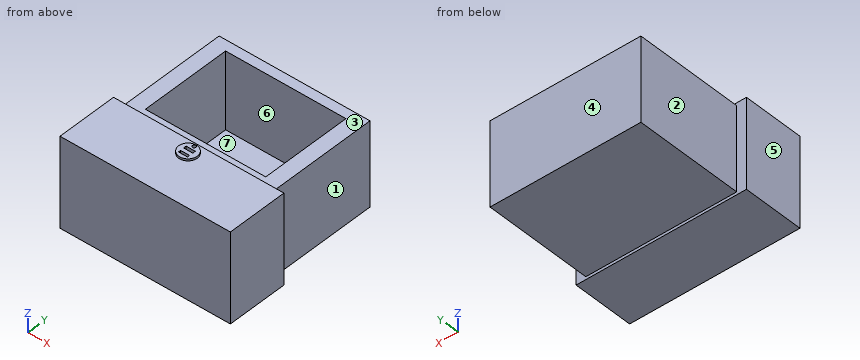
from build123d import *

# Parameters (mm, degrees)
F0_W      = 236.721322
F0_H      = 124.82763
F1_DEPTH  = 84.582
F2_W      = 209.650278
F2_H      = 117.007106
F3_DEPTH  = 151.384
F4_W      = 167.194322
F4_H      = 126.676479
F5_DEPTH  = 106.934
F6_R      = 12.932429
F7_DEPTH  = 2.794
F8_W      = 12.893153
F8_H      = 4.004114
F8_W_2    = 12.566442
F8_H_2    = 3.328527
F9_DEPTH  = 14.732
F10_R     = 2.422057
F11_DEPTH = 25.4


with BuildPart() as f1:
    # F0 (on Front) → F1 (new body)
    with BuildSketch(Plane.XZ):
        Rectangle(F0_W, F0_H)
    extrude(amount=F1_DEPTH)

    # F2 (on face) → F3 (join)
    with BuildSketch(Plane(origin=(0, 0, 0), x_dir=(-1, 0, 0), z_dir=(0, 1, 0))):
        Rectangle(F2_W, F2_H)
    extrude(amount=F3_DEPTH)

    # F4 (on face) → F5 (cut)
    with BuildSketch(Plane.XY.offset(58.503553)):
        with Locations((0, 74.151702)):
            Rectangle(F4_W, F4_H)
    extrude(amount=-F5_DEPTH, mode=Mode.SUBTRACT)

    # F6 (on face) → F7 (join)
    with BuildSketch(Plane.XY.offset(62.413815)):
        with Locations((0, -16.961597)):
            Circle(F6_R)
    extrude(amount=F7_DEPTH)

    # F8 (on face) → F9 (cut)
    with BuildSketch(Plane.XY.offset(65.207815)):
        with Locations((-0.298541, -14.347668)):
            Rectangle(F8_W, F8_H)
        with Locations((-0.135185, -23.072623)):
            Rectangle(F8_W_2, F8_H_2)
    extrude(amount=-F9_DEPTH, mode=Mode.SUBTRACT)

    # F10 (on face) → F11 (cut)
    with BuildSketch(Plane.XY.offset(65.207815)):
        with Locations((0, -7.139143)):
            Circle(F10_R)
    extrude(amount=-F11_DEPTH, mode=Mode.SUBTRACT)


solid = f1.part
Could you check a few things on this model? Use its own coordinates, in mm. Face numbers are marked on the shaded views. A direction names the side the tool comes from. Give positions to 0.01 mm unless a question says otherwise; leave off trailing zeros. Write each loop counter-clockwise with the first axis right and the second up, starting at its lowest first coordinate (ties: lowest second). Pieces come first, ordered by that corner, then holes. Notation, with made-up numbers: (-28, -5) -> (9, -5) arc R18 cw to (9, 19) -> close; hole circle Ø8 at (59, 26.5). An arc over 180 degrees is marked (long way). Answer as CSV lines item,"result". Start each with the question number.
(1) If we mould it in two halves opening along Y, with no side actions, what happens to the marked faces 4, 5, 6 and 7? For each: +Y half, -Y half, draft (parallel to the pull), parting line (faces both ways), or undercut.
(2) If we section it at A-A, the plane z = 20.5: Write out the boundary of the cut face in (x, y).
(3) Which directions (+Z, -Z, +X, -X, +Y, -Y) give clear straight access to the entire face, cutting with the end or side of a thin tool? Please do the marked faces 1, 2 and 3.
(4) I'm going to push flat-ended pins straight in: pin 1 Ø1.5 at (y, z) = (36.5, 16) entering from -X; pin 2 Ø4 at (x, y) = (48.5, 81) entering from +Z; pin 3 Ø2.5 at (x, y) = (1, -7.5) entering from +Z. Where does each tip first touch, or does it pass through?
(5) If we section it at B-B, the plane x = 31: Write out the boundary of the cut face in (y, z), and give its area (3 significant figures).
(6) Please list where these lines run through material, in increasing order: line 1 (Y direction, x = 0, z = 55); line 2 (X direction, y = 121.5, z = 31.5); line 3 (Y direction, x = 8.5, z = 18).
(7) If we section it at C-C, the plane y = 114.5: Write out the boundary of the cut face in (x, z), and give its area (3 significant figures).
Answer list:
1,face 4,"+Y half"
1,face 5,"draft"
1,face 6,"undercut"
1,face 7,"undercut"
2,outline,"(-118.36, -84.58) -> (118.36, -84.58) -> (118.36, 0) -> (104.83, 0) -> (104.83, 151.38) -> (-104.83, 151.38) -> (-104.83, 0) -> (-118.36, 0) -> close; hole (-83.6, 10.81) -> (83.6, 10.81) -> (83.6, 137.49) -> (-83.6, 137.49) -> close"
3,face 1,"+Z, -Z, +X, +Y"
3,face 2,"+Z, -Z, -X, +Y"
3,face 3,"+Z, +X, -X, +Y"
4,pin 1,"x = -104.83"
4,pin 2,"z = -48.43"
4,pin 3,"z = 39.81"
5,outline,"(-84.58, -62.41) -> (0, -62.41) -> (0, -58.5) -> (151.38, -58.5) -> (151.38, 58.5) -> (137.49, 58.5) -> (137.49, -48.43) -> (10.81, -48.43) -> (10.81, 58.5) -> (0, 58.5) -> (0, 62.41) -> (-84.58, 62.41) -> close"
5,area,"14,700 mm^2"
6,line 1,"-84.58 to -24.74, -21.41 to -16.35, -12.35 to -9.56, -4.72 to 10.81, 137.49 to 151.38"
6,line 2,"-104.83 to -83.6, 83.6 to 104.83"
6,line 3,"-84.58 to 10.81, 137.49 to 151.38"
7,outline,"(-104.83, -58.5) -> (104.83, -58.5) -> (104.83, 58.5) -> (83.6, 58.5) -> (83.6, -48.43) -> (-83.6, -48.43) -> (-83.6, 58.5) -> (-104.83, 58.5) -> close"
7,area,"6,650 mm^2"
